Work out the finished part from the listing and answer in its coordinate system (mm). Face numbers are marked on the shaded views. A direction names the side the tool comes from. Coordinates: 2 decimals unless noted, no trailing zeros. Write each loop counter-clockwise with the first axis right and the second up, starting at its lowest first coordinate (ties: lowest second). Pieces come first, ordered by that corner, then holes. Notation, with made-up numbers: (56.5, -22) - (69.5, -22) arc R12 ccw to (69.5, -16) - close; hole circle Ø4 at (77.25, 46). An arc over 180 degrees is marked (long way). Use one line per item in the form item = value. Start each with the question number.
Item 1: For the marked faces 1, 2 and 3, determine the directions among +Z, -Z, +X, -X, +Y, -Y from which every point of the face is accessible in a straight line to the end or side of a thin tool.
Item 2: A cutting plane is placed at A-A (x = 32). Write down the section's boundary in (y, z), then the cut area to 3 significant figures.
Item 3: A cutting plane is placed at B-B (z = 9.75). Write down the section's boundary in (x, y), then the cut area to 3 significant figures.
Item 4: A cutting plane is placed at D-D (z = 3.75). Write down the section's boundary in (x, y).
Item 5: A cutting plane is placed at C-C (y = 3.5). Write down the section's boundary in (x, z).
Item 6: Given pin 1 (4.5 mm diameter, centred on x = 10, y = 6.5, fed in from -Z); pin 2 (8 mm diameter, centred on x = 10, y = 6.5, fed in from +Z); pin 3 (5.5 mm diameter, centred on y = 7, z = 2, fed in from -X); pin 4 (6 mm diameter, centred on x = 10.5, z = 3.5, fed in from +Y), each flat-ended and moving along its own axis, determine where each tip first touches the part or whether it passes through.
Item 7: Determine the mould class of the marked faces 4, 5 and 6 for opening direction Y: released by +Y, released by -Y, zero draft, split by the parting line, or undercut.
Item 8: Consider probe 1 along Y at (x, z) = (32, 2.75); probe 2 along Y at (x, z) = (10, 8.5); probe 3 along Z at (x, y) = (10.5, 2.5). Determine where each line is inside the solid, lowest interval first.
from build123d import *

# Parameters (mm, degrees)
SKETCH_1_W                   = 35.5
SKETCH_1_H                   = 17.5
EXTRUDE_1_DEPTH              = 12
SKETCH_2_W                   = 18.5
SKETCH_2_H                   = 4.5
CUT_EXTRUDE_1_DEPTH          = 42.35819145
SKETCH_3_R                   = 5
CUT_EXTRUDE_2_DEPTH          = 4.5
HOLE_WIZARD_M3_1_D           = 3.6
HOLE_WIZARD_M3_1_CBORE_D     = 6.5
HOLE_WIZARD_M3_1_CBORE_DEPTH = 3
SKETCH_8_R                   = 2.5
CUT_EXTRUDE_3_DEPTH          = 41.283371259
SKETCH_10_W                  = 17
SKETCH_10_H                  = 13
CUT_EXTRUDE_4_DEPTH          = 5


with BuildPart() as part:
    # 草图1 → 凸台-拉伸1 (new body)
    with BuildSketch(Plane.XY):
        with Locations((17.75, 8.75)):
            Rectangle(SKETCH_1_W, SKETCH_1_H)
    extrude(amount=EXTRUDE_1_DEPTH)

    # 草图2 → 切除-拉伸1 (cut, through all)
    with BuildSketch(Plane.XY.offset(12)):
        with Locations((9.25, 15.25)):
            Rectangle(SKETCH_2_W, SKETCH_2_H)
    extrude(amount=-CUT_EXTRUDE_1_DEPTH, mode=Mode.SUBTRACT)

    # 草图3 → 切除-拉伸2 (cut)
    with BuildSketch(Plane.XY.offset(12)):
        with Locations((10, 6.5)):
            Circle(SKETCH_3_R)
    extrude(amount=-CUT_EXTRUDE_2_DEPTH, mode=Mode.SUBTRACT)

    # M3 六角凹头螺钉的柱形沉头孔1 (through all)
    with Locations(Plane.XY.offset(12)):
        with Locations((22, 14), (32, 3.5)):
            CounterBoreHole(HOLE_WIZARD_M3_1_D / 2, HOLE_WIZARD_M3_1_CBORE_D / 2, HOLE_WIZARD_M3_1_CBORE_DEPTH)

    # 草图8 → 切除-拉伸3 (cut, through all)
    with BuildSketch(Plane.XY.offset(7.5)):
        with Locations((10, 6.5)):
            Circle(SKETCH_8_R)
    extrude(amount=-CUT_EXTRUDE_3_DEPTH, mode=Mode.SUBTRACT)

    # 草图10 → 切除-拉伸4 (cut)
    with BuildSketch(Plane(origin=(0, 0, 0), x_dir=(-1, 0, 0), z_dir=(0, 0, -1))):
        with Locations((-8.5, 6.5)):
            Rectangle(SKETCH_10_W, SKETCH_10_H)
    extrude(amount=-CUT_EXTRUDE_4_DEPTH, mode=Mode.SUBTRACT)


solid = part.part
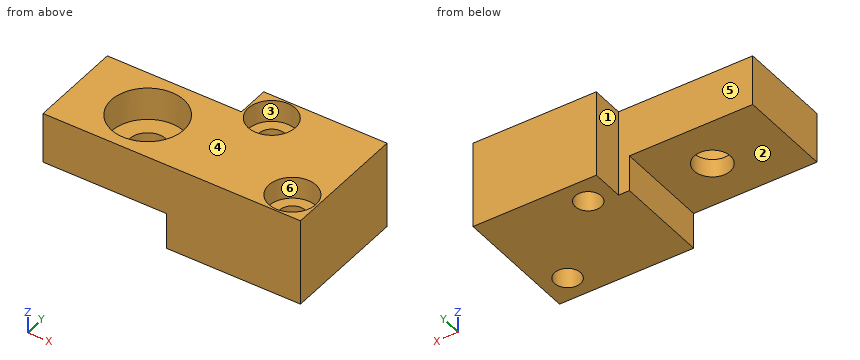
Answer:
q1.face_1 = +Z, -Z, -X, +Y
q1.face_2 = -Z, -X, +Y, -Y
q1.face_3 = +Z
q2.outline = (0, 0) - (1.7, 0) - (1.7, 9) - (0.25, 9) - (0.25, 12) - (0, 12) - close; (5.3, 0) - (17.5, 0) - (17.5, 12) - (6.75, 12) - (6.75, 9) - (5.3, 9) - close
q2.area = 158 mm²
q3.outline = (0, 0) - (35.5, 0) - (35.5, 17.5) - (18.5, 17.5) - (18.5, 13) - (0, 13) - close; hole circle Ø10 at (10, 6.5); hole circle Ø6.5 at (22, 14); hole circle Ø6.5 at (32, 3.5)
q3.area = 393 mm²
q4.outline = (17, 0) - (35.5, 0) - (35.5, 17.5) - (18.5, 17.5) - (18.5, 13) - (17, 13) - close; hole circle Ø3.6 at (22, 14); hole circle Ø3.6 at (32, 3.5)
q5.outline = (0, 5) - (17, 5) - (17, 0) - (30.2, 0) - (30.2, 9) - (28.75, 9) - (28.75, 12) - (14, 12) - (14, 7.5) - (6, 7.5) - (6, 12) - (0, 12) - close; (33.8, 0) - (35.5, 0) - (35.5, 12) - (35.25, 12) - (35.25, 9) - (33.8, 9) - close
q6.pin_1 = through
q6.pin_2 = 7.5
q6.pin_3 = 17
q6.pin_4 = 13
q7.face_4 = zero draft
q7.face_5 = released by +Y
q7.face_6 = undercut
q8.probe_1 = 0 to 1.7, 5.3 to 17.5
q8.probe_2 = 0 to 1.5, 11.5 to 13
q8.probe_3 = 5 to 7.5
